Design review of the part built by this model. Coordinates are the model's own, in mm. Face numbers are marked on the shaded views. A direction names the side the tool comes from. Give positions to 0.01 mm unless a question says otherwise; leave off trailing zeros. Write each loop counter-clockwise with the first axis right and the second up, starting at its lowest first coordinate (ties: lowest second). Pieces come first, ordered by that corner, then holes.
```python
from build123d import *

# Parameters (mm, degrees)
BOSS_EXTRUDE1_DEPTH = 74
SKETCH2_R           = 1.5
CUT_EXTRUDE1_DEPTH  = 1
SKETCH4_W           = 60
SKETCH4_H           = 34
CUT_EXTRUDE2_DEPTH  = 1
SKETCH6_W           = 7
SKETCH6_H           = 34
CUT_EXTRUDE3_DEPTH  = 1
SKETCH7_R           = 1.5
CUT_EXTRUDE4_DEPTH  = 1
SKETCH8_R           = 4
SKETCH8_R_2         = 1.5
CUT_EXTRUDE5_DEPTH  = 1
SKETCH9_W           = 19.5
SKETCH9_H           = 7
CUT_EXTRUDE6_DEPTH  = 1
FILLET1_R           = 2


with BuildPart() as part:
    # Sketch1 → Boss-Extrude1 (new body)
    with BuildSketch(Plane.XY):
        Polygon((-68.212386303, 4.586111111), (-68.212386303, -28.413888889), (-26.212386303, -28.413888889), (-26.212386303, 4.586111111), (-25.212386303, 4.586111111), (-25.212386303, -29.413888889), (-69.212386303, -29.413888889), (-69.212386303, 4.586111111), align=None)
    extrude(amount=BOSS_EXTRUDE1_DEPTH)

    # Sketch2 → Cut-Extrude1 (cut)
    with BuildSketch(Plane(origin=(-25.212386303, 0, 0), x_dir=(0, 0, -1), z_dir=(1, 0, 0))):
        with Locations((-3, -1.913888889)):
            Circle(SKETCH2_R)
        with Locations((-71, -1.913888889)):
            Circle(SKETCH2_R)
        with Locations((-71, -17.913888889)):
            Circle(SKETCH2_R)
        with Locations((-3, -17.913888889)):
            Circle(SKETCH2_R)
    extrude(amount=-CUT_EXTRUDE1_DEPTH, mode=Mode.SUBTRACT)

    # Sketch4 → Cut-Extrude2 (cut)
    with BuildSketch(Plane(origin=(-25.212386303, 0, 0), x_dir=(0, 0, -1), z_dir=(1, 0, 0))):
        with Locations((-37, -12.413888889)):
            Rectangle(SKETCH4_W, SKETCH4_H)
    extrude(amount=-CUT_EXTRUDE2_DEPTH, mode=Mode.SUBTRACT)

    # Sketch6 → Cut-Extrude3 (cut)
    with BuildSketch(Plane.ZY.offset(69.212386303)):
        with Locations((3.5, -12.413888889)):
            Rectangle(SKETCH6_W, SKETCH6_H)
        with Locations((70.5, -12.413888889)):
            Rectangle(SKETCH6_W, SKETCH6_H)
    extrude(amount=-CUT_EXTRUDE3_DEPTH, mode=Mode.SUBTRACT)

    # Sketch7 → Cut-Extrude4 (cut)
    with BuildSketch(Plane.ZY.offset(69.212386303)):
        with Locations((58, -9.413888889)):
            Circle(SKETCH7_R)
        with Locations((26, -9.413888889)):
            Circle(SKETCH7_R)
    extrude(amount=-CUT_EXTRUDE4_DEPTH, mode=Mode.SUBTRACT)

    # Sketch8 → Cut-Extrude5 (cut)
    with BuildSketch(Plane(origin=(0, -29.413888889, 0), x_dir=(-1, 0, 0), z_dir=(0, -1, 0))):
        with Locations((39.212386303, -37)):
            Circle(SKETCH8_R)
        with Locations((39.212386303, -29)):
            Circle(SKETCH8_R_2)
        with Locations((47.212386303, -37)):
            Circle(SKETCH8_R_2)
        with Locations((39.212386303, -45)):
            Circle(SKETCH8_R_2)
        with Locations((31.212386303, -37)):
            Circle(SKETCH8_R_2)
        with Locations((31.212386303, -21)):
            Circle(SKETCH8_R_2)
        with Locations((39.212386303, -13)):
            Circle(SKETCH8_R_2)
        with Locations((47.212386303, -21)):
            Circle(SKETCH8_R_2)
        with Locations((39.212386303, -21)):
            Circle(SKETCH8_R)
        with Locations((39.212386303, -61)):
            Circle(SKETCH8_R_2)
        with Locations((39.212386303, -53)):
            Circle(SKETCH8_R)
        with Locations((47.212386303, -53)):
            Circle(SKETCH8_R_2)
        with Locations((31.212386303, -53)):
            Circle(SKETCH8_R_2)
    extrude(amount=-CUT_EXTRUDE5_DEPTH, mode=Mode.SUBTRACT)

    # Sketch9 → Cut-Extrude6 (cut)
    with BuildSketch(Plane.XZ.offset(29.413888889)):
        with Locations((-58.462386303, 3.5)):
            Rectangle(SKETCH9_W, SKETCH9_H)
        with Locations((-58.462386303, 70.5)):
            Rectangle(SKETCH9_W, SKETCH9_H)
    extrude(amount=-CUT_EXTRUDE6_DEPTH, mode=Mode.SUBTRACT)

    # Fillet1
    fillet1_edges = [part.edges().sort_by_distance(p)[0] for p in [
        (-48.712386303, -28.913888889, 0),
        (-25.712386303, 4.586111111, 74),
        (-48.712386303, -28.913888889, 74),
        (-68.712386303, 4.586111111, 7),
        (-68.212386303, -28.413888889, 37),
        (-69.212386303, -29.413888889, 37),
        (-68.712386303, 4.586111111, 67),
        (-25.712386303, 4.586111111, 0),
    ]]
    fillet(fillet1_edges, radius=FILLET1_R)


solid = part.part
```
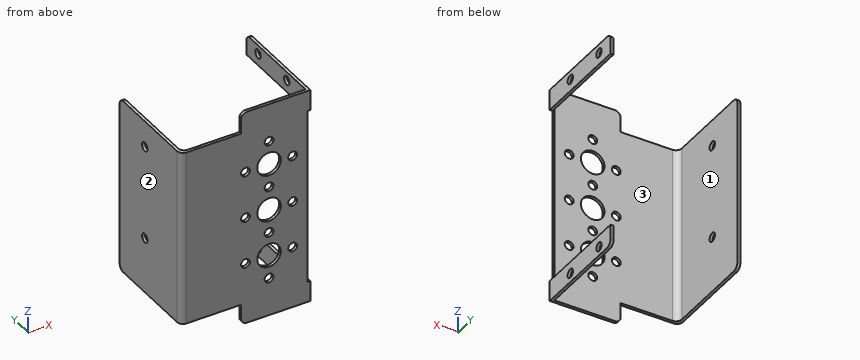
(1) Consider section D-D, the plane z = 21. Give the boundary of the cut face in (x, y), then the cut area to 3 significant figures.
Resolved:
outline: (-69.21, -27.41) arc R2 ccw to (-67.21, -29.41) - (-48.71, -29.41) - (-48.71, -28.41) - (-66.21, -28.41) arc R2 cw to (-68.21, -26.41) - (-68.21, 4.59) - (-69.21, 4.59) - close; (-45.71, -29.41) - (-43.21, -29.41) - (-43.21, -28.41) - (-45.71, -28.41) - close; (-35.21, -29.41) - (-32.71, -29.41) - (-32.71, -28.41) - (-35.21, -28.41) - close; (-29.71, -29.41) - (-26.21, -29.41) - (-26.21, -28.41) - (-29.71, -28.41) - close
area: 62.0 mm2
(2) Consider section A-A, the plane y = -14. Give the boundary of the cut face in (x, z).
Resolved:
outline: (-69.21, 7) - (-68.21, 7) - (-68.21, 67) - (-69.21, 67) - close; (-26.21, 0) - (-25.21, 0) - (-25.21, 7) - (-26.21, 7) - close; (-26.21, 67) - (-25.21, 67) - (-25.21, 74) - (-26.21, 74) - close
(3) Consider section C-C, the plane z = 3. Give the boundary of the cut face in (x, y), then the cut area to 3 significant figures.
Resolved:
outline: (-48.71, -29.41) - (-25.21, -29.41) - (-25.21, -19.41) - (-26.21, -19.41) - (-26.21, -28.41) - (-48.71, -28.41) - close; (-26.21, -16.41) - (-25.21, -16.41) - (-25.21, -3.41) - (-26.21, -3.41) - close; (-26.21, -0.41) - (-25.21, -0.41) - (-25.21, 4.59) - (-26.21, 4.59) - close
area: 50.5 mm2
(4) To check wall thickness, follow L1, parallel to Y at x = -25.5, z = 3; L2, parallel to X at y = -7.5, z = 59.5; L3, parallel to X at y = -29, z = 37. State the ranges of each line that lie inside material, in increasing order.
Resolved:
L1: y = -29.41 to -19.41, -16.41 to -3.41, -0.41 to 4.59
L2: x = -69.21 to -68.21
L3: x = -68.43 to -48.71, -45.71 to -43.21, -35.21 to -32.71, -29.71 to -26.21
(5) Consider section B-B, the plane z = 29. Give the boundary of the cut face in (x, y), then the cut area to 3 significant figures.
Resolved:
outline: (-69.21, -27.41) arc R2 ccw to (-67.21, -29.41) - (-40.71, -29.41) - (-40.71, -28.41) - (-66.21, -28.41) arc R2 cw to (-68.21, -26.41) - (-68.21, 4.59) - (-69.21, 4.59) - close; (-37.71, -29.41) - (-26.21, -29.41) - (-26.21, -28.41) - (-37.71, -28.41) - close
area: 73.0 mm2
(6) Clearance check with flat-ended pins moving along their axes: P1, Ø1.8, axis at y = -1.91, z = 3, coming from the -X side; P2, Ø6, axis at y = -8.5, z = 11.5, coming from the +X side; P3, Ø6, axis at x = -38.5, z = 22.5, coming from the +Y side; P4, Ø4, axis at y = -1.91, z = 71, coming from the -X side. State where each tip first meets the part, or that it passes through.
Resolved:
P1: passes through
P2: stops at x = -68.21
P3: stops at y = -28.41
P4: stops at x = -26.21
(7) Tool access review of the marked faces 1, 2 and 3: name each direction out of +Z, -Z, +X, -X, +Y, -Y from which nothing blocks a thin tool from reaching the whole face with its end or side.
Resolved:
face 1: +Z, -Z, +X, +Y
face 2: +Z, -Z, -X, +Y, -Y
face 3: +Z, -Z, +Y
